```python
from build123d import *

# Parameters (mm, degrees)
F1_DEPTH = 6.35
F2_DEPTH = 6.35
F4_D     = 25.4
F0_R     = 14.2875
F5_DEPTH = 6.35


with BuildPart() as f1:
    # F0 (on Right) → F1 (new body)
    with BuildSketch(Plane.YZ):
        with BuildLine():
            ThreePointArc((-2.099991, -204.28443), (-2.100104, -204.39856), (-2.100445, -204.512689))
            Line((-2.100445, -204.512689), (18.158056, -77.147721))
            ThreePointArc((18.158056, -77.147721), (49.128885, -21.909255), (108.5466, 0))
            Line((108.5466, 0), (165.976715, 0))
            ThreePointArc((165.976715, 0), (198.077363, -8.676495), (221.435985, -32.343096))
            Line((221.435985, -32.343096), (249.324016, -81.635659))
            ThreePointArc((249.324016, -81.635659), (253.014213, -83.19258), (255.459351, -80.020378))
            Line((255.459351, -80.020378), (255.459351, -2.815202))
            Line((255.459351, -2.815202), (263.697012, 102.492085))
            ThreePointArc((263.697012, 102.492085), (261.769548, 105.424616), (258.449354, 104.288324))
            Line((258.449354, 104.288324), (227.64977, 57.433632))
            ThreePointArc((227.64977, 57.433632), (206.146196, 39.32667), (178.240132, 35.932943))
            Line((178.240132, 35.932943), (-21.036066, 69.812165))
            ThreePointArc((-21.036066, 69.812165), (-44.087909, 64.971566), (-57.640454, 45.706379))
            Line((-57.640454, 45.706379), (-113.891336, -186.494963))
            ThreePointArc((-113.891336, -186.494963), (-50.404443, -147.685468), (-2.099991, -204.28443))
        make_face()
    extrude(amount=F1_DEPTH)

    # F0 (on Right) → F2 (join)
    with BuildSketch(Plane.YZ):
        with BuildLine():
            ThreePointArc((-2.099991, -204.28443), (-2.100104, -204.39856), (-2.100445, -204.512689))
            Line((-2.100445, -204.512689), (18.158056, -77.147721))
            ThreePointArc((18.158056, -77.147721), (49.128885, -21.909255), (108.5466, 0))
            Line((108.5466, 0), (165.976715, 0))
            ThreePointArc((165.976715, 0), (198.077363, -8.676495), (221.435985, -32.343096))
            Line((221.435985, -32.343096), (249.324016, -81.635659))
            ThreePointArc((249.324016, -81.635659), (253.014213, -83.19258), (255.459351, -80.020378))
            Line((255.459351, -80.020378), (255.459351, -2.815202))
            Line((255.459351, -2.815202), (263.697012, 102.492085))
            ThreePointArc((263.697012, 102.492085), (261.769548, 105.424616), (258.449354, 104.288324))
            Line((258.449354, 104.288324), (227.64977, 57.433632))
            ThreePointArc((227.64977, 57.433632), (206.146196, 39.32667), (178.240132, 35.932943))
            Line((178.240132, 35.932943), (-21.036066, 69.812165))
            ThreePointArc((-21.036066, 69.812165), (-44.087909, 64.971566), (-57.640454, 45.706379))
            Line((-57.640454, 45.706379), (-113.891336, -186.494963))
            ThreePointArc((-113.891336, -186.494963), (-50.404443, -147.685468), (-2.099991, -204.28443))
        make_face()
    extrude(amount=F2_DEPTH)

    # F4 (through all)
    with Locations(Plane.YZ.offset(6.35)):
        with Locations((236.524433, 16.445378)):
            Hole(F4_D / 2)

    # F0 (on Right) → F5 (join)
    with BuildSketch(Plane.YZ):
        with BuildLine():
            ThreePointArc((-113.891336, -186.494963), (-68.530434, -260.865344), (-2.100445, -204.512689))
            ThreePointArc((-2.100445, -204.512689), (-2.100104, -204.39856), (-2.099991, -204.28443))
            ThreePointArc((-2.099991, -204.28443), (-50.404443, -147.685468), (-113.891336, -186.494963))
        make_face()
        with Locations((-59.411091, -204.28443)):
            Circle(F0_R, mode=Mode.SUBTRACT)
    extrude(amount=F5_DEPTH)


solid = f1.part
```
Source: CAD feature listing. Evaluate the final solid. Frame: model axes, mm. A direction names the side the tool comes from. Round coordinates to 2 decimals unless told otherwise and drop trailing zeros. Loops run counter-clockwise (first coordinate to the right, second up) from the corner with the lowest first, then second, coordinate; pieces in that order, holes last.
1. Contact query for flat-ended pins moving along their axis: pin 1 (3 mm diameter, centred on x = 2, z = 18, fed in from +Y); pin 2 (3 mm diameter, centred on x = 5.5, z = -24, fed in from +Y); pin 3 (1 mm diameter, centred on x = 5.5, z = -129.5, fed in from -Y); pin 4 (6 mm diameter, centred on y = 6.5, z = -56.5, fed in from -X). Output: stop coordinate, or through.
2. Mould query, pull axis Z, two halves, no side actions, for faces 4 (the flat face through (3.131, -85.372, -68.769)), 5 (the cylindrical face through (3.131, 48.443, -22.5)), 6 (the cylindrical face through (3.131, 249.212, 17.004)). Classes: released by +Z, released by -Z, zero draft, split by the parting line, or undercut.
3. Section query A-A on z = -13.5. Output: boundary loops of the cut face in (x, y), and give its area (3 significant figures).
4. Section query D-D on z = -126.5. Output: boundary loops of the cut face in (x, y), and give its area (3 significant figures).
5. Ray query, L1, parallel to Y at x = 5, z = 23; L2, parallel to Y at x = 0.5, z = 10.5; L3, parallel to Z at x = 5.5, y = -52. Return the intervals inside material, ascending.
6. Section query B-B on x = 5.25. Output: boundary loops of the cut face in (y, z) (1 decimal).
7. Section query C-C on y = 125.5. Output: boundary loops of the cut face in (x, z), and give its area (3 significant figures).
8. Access query for faces 1 (the flat face through (3.13, 259.52, 49.1)), 2 (the cylindrical face through (3.13, 197.67, -8.44)), 3 (the flat face through (3.131, 243.265, 81.189)). Directions: +Z, -Z, +X, -X, +Y, -Y. A direction counts if a zero-diameter tool reaches every point of the face in a straight line with its end or side. Return the directions, or none.
Answers below:
1. pin 1: stops at y = 257.2
1. pin 2: stops at y = 255.46
1. pin 3: stops at y = -100.21
1. pin 4: stops at x = 0
2. face 4: released by +Z
2. face 5: released by -Z
2. face 6: undercut
3. outline: (0, -71.98) - (6.35, -71.98) - (6.35, 60.7) - (0, 60.7) - close; (0, 205.2) - (6.35, 205.2) - (6.35, 255.46) - (0, 255.46) - close
3. area: 1,160 mm2
4. outline: (0, -99.36) - (6.35, -99.36) - (6.35, 10.31) - (0, 10.31) - close
4. area: 696 mm2
5. L1: y = -63.14 to 225.65, 247.4 to 257.48
5. L2: y = -66.17 to 225.3, 247.75 to 256.5
5. L3: z = -261.11 to -216.5, -192.07 to 57.57
6. outline: (-113.9, -186.5) arc R57.3 ccw (long way) to (-2.1, -204.5) - (18.2, -77.1) arc R91.5 cw to (108.5, 0) - (166, 0) arc R63.7 cw to (221.4, -32.3) - (249.3, -81.6) arc R3.3 ccw to (255.5, -80) - (255.5, -2.8) - (263.7, 102.5) arc R2.9 ccw to (258.4, 104.3) - (227.6, 57.4) arc R49.3 cw to (178.2, 35.9) - (-21, 69.8) arc R32.1 ccw to (-57.6, 45.7) - close; hole circle Ø28.6 at (-59.4, -204.3); hole circle Ø25.4 at (236.5, 16.4)
7. outline: (0, 0) - (6.35, 0) - (6.35, 44.9) - (0, 44.9) - close
7. area: 285 mm2
8. face 1: -Z, +X, -X, +Y
8. face 2: -Z, +X, -X
8. face 3: +Z, +X, -X
